Design review of the part built by this model. Coordinates are the model's own, in mm. Face numbers are marked on the shaded views. Round coordinates to 2 decimals unless told otherwise and drop trailing zeros. Loops run counter-clockwise (first coordinate to the right, second up) from the corner with the lowest first, then second, coordinate; pieces in that order, holes last. Notation, with made-up numbers: (68, 84) - (82, 84) arc R19 cw to (82, 110) - close; hole circle Ø7 at (-16.75, 85). An arc over 180 degrees is marked (long way). Use one line per item in the form item = value. Start each with the question number.
(1) For pin 1 (1.9 mm diameter, centred on y = 2, z = -36, fed in from -X); pin 2 (3 mm diameter, centred on y = 409.5, z = -21.5, fed in from +X); pin 3 (12 mm diameter, centred on y = 224, z = -34.5, fed in from +X), all flat-tipped, find the tip position at first contact; note any pin that passes through.
(2) We need section B-B, the plane x = -16. Write out the cut boundary in (y, z).
(3) We need section A-A, the plane z = 0. Write out the cut boundary in (x, y), then the cut area to 3 significant figures.
(4) Wall thickness on probe 1 along Z at (x, y) = (0, 180.5); probe 2 along X at (y, z) = (208, 2.5): over which ranges is each line inside the solid? List them lowest first. Write a range as [from, to].
(5) We need section C-C, the plane y = 130. Write out the cut boundary in (x, z), then the cut area to 3 significant figures.
(6) The part is to be moulded in two halves that separate along Z. For the marked faces 1 and 2, say which applies: released by +Z, released by -Z, zero draft, split by the parting line, or undercut.
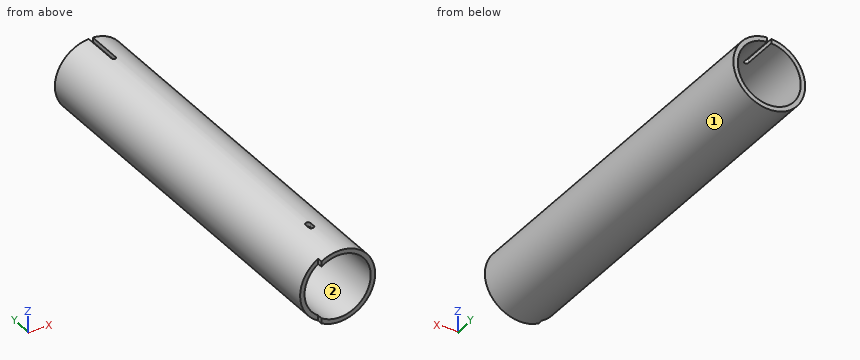
Autodesk Inventor part; units mm, degrees
ref_plane "Work Plane1" through (0, 0, 44.45) normal (0, 0, 1) x (1, 0, 0)
ref_plane "YZ Plane" through (0, 0, 0) normal (1, 0, 0) x (0, 1, 0)
ref_plane "XZ Plane" through (0, 0, 0) normal (0, 1, 0) x (-1, 0, 0)
sketch "Sketch1" plane through (0, 0, 0) normal (0, 1, 0) x (-1, 0, 0)
  circle A0 centre (0, 0) radius 44.45
  circle A1 centre (0, 0) radius 38.9636
  dimension "d0" = 88.9
  dimension "d1" = 5.4864
extrude "Extrusion1" add sketch "Sketch1" along normal blind 481.33
ref_plane "Work Plane1" through (0, 0, 44.45) normal (0, 0, 1) x (1, 0, 0)
sketch "Sketch2" plane through (0, 0, 44.45) normal (0, 0, 1) x (1, 0, 0)
  arc A0 (-2.54, 436.88) -> (2.54, 436.88) centre (0, 436.88) ccw
  line L0 (44.45, 481.33) -> (-44.45, 481.33)
  line L1 (-2.54, 436.88) -> (-2.54, 481.33)
  line L2 (2.54, 436.88) -> (2.54, 481.33)
  point P0 (0, 0)
  dimension "d5" = 44.45
  dimension "d6" = 5.08
extrude "Extrusion2" cut sketch "Sketch2" against normal blind 25.4
sketch "Sketch4" plane through (0, 0, 44.45) normal (0, 0, 1) x (1, 0, 0)
  line L0 (0, 54.102) -> (0, 60.452) construction
  line L1 (3.175, 54.102) -> (3.175, 60.452)
  line L2 (-3.175, 60.452) -> (-3.175, 54.102)
  arc A0 (-3.175, 54.102) -> (3.175, 54.102) centre (0, 54.102) ccw
  arc A1 (3.175, 60.452) -> (-3.175, 60.452) centre (0, 60.452) ccw
  point P0 (0, 0)
  point P1 (0, 57.277)
  dimension "d18" = 6.35
  dimension "d19" = 6.35
  dimension "d20" = 54.102
extrude "Extrusion3" cut sketch "Sketch4" against normal blind 25.4
sketch "Sketch5" plane through (0, 0, 0) normal (0, -1, 0) x (1, 0, 0)
  circle A0 centre (0, 0) radius 44.45
  line L0 (-22.098, 38.5679) -> (-22.098, -38.5679)
  point P0 (-44.45, 0)
  dimension "d23" = 22.352
extrude "Extrusion4" cut sketch "Sketch5" against normal blind 6.35 contours L0 A0 picked at (-24.6172, 11.037)
properties part number "mast_paper"
Data:
q1.pin_1 = -22.1
q1.pin_2 = 39.7
q1.pin_3 = 34.11
q2.outline = (0, -41.47) - (481.33, -41.47) - (481.33, -35.53) - (0, -35.53) - close; (0, 35.53) - (481.33, 35.53) - (481.33, 41.47) - (0, 41.47) - close
q3.outline = (-44.45, 6.35) - (-38.96, 6.35) - (-38.96, 481.33) - (-44.45, 481.33) - close; (38.96, 0) - (44.45, 0) - (44.45, 481.33) - (38.96, 481.33) - close
q3.area = 5,250 mm^2
q4.probe_1 = [-44.45, -38.96], [38.96, 44.45]
q4.probe_2 = [-44.38, -38.88], [38.88, 44.38]
q5.outline = circle Ø88.9 at (0, 0); hole circle Ø77.93 at (0, 0)
q5.area = 1,440 mm^2
q6.face_1 = split by the parting line
q6.face_2 = undercut
